```python
from build123d import *

# Parameters (mm, degrees)
F1_DEPTH = 5
F2_W     = 34.5
F2_H     = 5
F3_DEPTH = 25
F4_R     = 2
F5_DEPTH = 25


with BuildPart() as f1:
    # F0 (on Front) → F1 (new body)
    with BuildSketch(Plane.XZ):
        with BuildLine():
            Line((-105.5, 20.25), (-105.5, 35.25))
            Line((-105.5, 35.25), (-86.5, 35.25))
            Line((-86.5, 35.25), (-86.5, 49.25))
            ThreePointArc((-86.5, 49.25), (-91.344095, 56.609669), (-98.5, 61.75))
            ThreePointArc((-98.5, 61.75), (-119.628789, 45.963308), (-125.5, 20.25))
            Line((-125.5, 20.25), (-105.5, 20.25))
        make_face()
        Polygon((-86.5, 35.25), (-105.5, 35.25), (-105.5, 20.25), (-105.5, -35.25), (105.5, -35.25), (105.5, 20.25), (105.5, 35.25), (86.5, 35.25), align=None)
        with BuildLine():
            Line((86.5, 49.25), (86.5, 35.25))
            Line((86.5, 35.25), (105.5, 35.25))
            Line((105.5, 35.25), (105.5, 20.25))
            Line((105.5, 20.25), (125.5, 20.25))
            ThreePointArc((125.5, 20.25), (119.628789, 45.963308), (98.5, 61.75))
            ThreePointArc((98.5, 61.75), (91.344095, 56.609669), (86.5, 49.25))
        make_face()
    extrude(amount=F1_DEPTH)

    # F2 (on face) → F3 (cut)
    with BuildSketch(Plane.XZ.offset(5)):
        Polygon((125.5, 20.25), (70.5, -35.25), (119.704917, -35.25), align=None)
        Polygon((-105.5, -35.25), (-11, -35.25), (-66.019693, 20.25), (-105.5, 20.25), align=None)
        with Locations((-13.75, 24.75)):
            Rectangle(F2_W, F2_H)
    extrude(amount=-F3_DEPTH, mode=Mode.SUBTRACT)

    # F4 (on face) → F5 (cut)
    with BuildSketch(Plane.XZ.offset(5)):
        with Locations((-99.5, 27.75)):
            Circle(F4_R)
        with Locations((99.5, 27.75)):
            Circle(F4_R)
    extrude(amount=-F5_DEPTH, mode=Mode.SUBTRACT)


solid = f1.part
```
The model under review builds one solid part; all positions refer to its coordinate system, in mm. A direction names the side the tool comes from. Coordinates: 2 decimals unless noted, no trailing zeros. Write each loop counter-clockwise with the first axis right and the second up, starting at its lowest first coordinate (ties: lowest second). Pieces come first, ordered by that corner, then holes. Notation, with made-up numbers: (15, 20) - (41, 20) arc R20 ccw to (41, 48) - close; hole circle Ø8 at (-33.5, 74.25). An arc over 180 degrees is marked (long way). Answer in a Markdown table with one row per item. Add a question column.
Q1. Draft analysis for pull direction Z (two halves, no side actions). For faces 1 (the face through (-86.5, -2, 42)), 2 (the face through (-31, -3, 25)), 3 (the face through (115, -2, 20.25)), state which applies: +Z half, -Z half, draft (parallel to the pull), parting line (faces both ways), or undercut.
Q2. For faces 4 (the face through (105.5, -2, 10)), 5 (the face through (-95, -3, 20.25)), 6 (the face through (1, -2, 35.25)), 7 (the face through (3.5, -3, 25)), 8 (the face through (29, -2, -35.25)), list the 3-axis set-ups (+Z, -Z, +X, -X, +Y, -Y) from which the entire face can be reached by the end or side of a thin tool; tool diameter is ignored.
Q3. Consider section D-D on z = -25. Give the boundary of the cut face in (x, y).
Q4. Clearance check with flat-ended pins moving along their axes: pin 1 (2.5 mm diameter, centred on y = -2, z = 44.5, fed in from +X); pin 2 (1.5 mm diameter, centred on x = -12, y = -3.5, fed in from +Z); pin 3 (2.5 mm diameter, centred on x = 120, y = -1.5, fed in from -Z). State where each tip first meets the part, or that it passes through.
Q5. Consider section B-B on z = 46. Give the boundary of the cut face in (x, y), then the cut area to 3 significant figures.
Q6. To check wall thickness, follow line 1 along Z through (x, y) = (-5, -1.8); line 2 along Z through (x, y) = (65.5, -2.4); line 3 along Z through (x, y) = (99.5, -3.45). State the ranges of each line that lie inside material, in increasing order. Write a range as from..to.
Q7. Consider section C-C on x = -79. Give the boundary of the cut face in (y, z).
Q8. Consider section A-A on y = -1.95. Give the boundary of the cut face in (x, z).
Answers below:
| question | item | result |
|---|---|---|
| 1 | face 1 | draft |
| 1 | face 2 | undercut |
| 1 | face 3 | -Z half |
| 2 | face 4 | -Z, +X, +Y, -Y |
| 2 | face 5 | -Z, -X, +Y, -Y |
| 2 | face 6 | +Z, +Y, -Y |
| 2 | face 7 | +Y, -Y |
| 2 | face 8 | -Z, +X, -X, +Y, -Y |
| 3 | outline | (-21.16, -5) - (80.66, -5) - (80.66, 0) - (-21.16, 0) - close |
| 4 | pin 1 | x = 121.24 |
| 4 | pin 2 | z = 35.25 |
| 4 | pin 3 | z = 20.25 |
| 5 | outline | (-119.6, -5) - (-86.5, -5) - (-86.5, 0) - (-119.6, 0) - close; (86.5, -5) - (119.6, -5) - (119.6, 0) - (86.5, 0) - close |
| 5 | area | 331 mm² |
| 6 | line 1 | -35.25..22.25, 27.25..35.25 |
| 6 | line 2 | -35.25..35.25 |
| 6 | line 3 | -5.99..25.75, 29.75..61.44 |
| 7 | outline | (-5, 20.25) - (0, 20.25) - (0, 35.25) - (-5, 35.25) - close |
| 8 | outline | (-125.5, 20.25) - (-66.02, 20.25) - (-11, -35.25) - (70.5, -35.25) - (105.5, 0.07) - (105.5, 20.25) - (125.5, 20.25) arc R38.22 ccw to (98.5, 61.75) arc R24.22 ccw to (86.5, 49.25) - (86.5, 35.25) - (-86.5, 35.25) - (-86.5, 49.25) arc R24.22 ccw to (-98.5, 61.75) arc R38.22 ccw to start; hole circle Ø4 at (-99.5, 27.75); hole (-31, 22.25) - (3.5, 22.25) - (3.5, 27.25) - (-31, 27.25) - close; hole circle Ø4 at (99.5, 27.75) |
